Part print with two shaded views. Sizes in mm from the minimum x, y, z corner. A direction names the side the tool comes from. Give positions to 0.01 mm unless a question says otherwise; leave off trailing zeros. Write each loop counter-clockwise with the first axis right and the second up, starting at its lowest first coordinate (ties: lowest second). Pieces come first, ordered by that corner, then holes. Notation, with made-up numbers: (55.25, 49.25) -> (86.25, 49.25) arc R15 cw to (86.25, 59.25) -> close; hole circle Ø1 at (9.5, 10.5). An arc over 180 degrees is marked (long way). Write item = value, one per line. Start each with the question number.
Q1. Saw through at C-C, the plane z = 3.5. List the corners of the cut face in (x, y), then the cut area to 3 significant figures.
Q2. Saw through at A-A, the plane x = 6. List the corners of the cut face in (y, z).
Q3. Drop flat-ended pins along their axis: P1, Ø3, axis at x = 4.5, z = 1, coming from the -Y side; P2, Ø2, axis at x = 8.5, z = 0.5, coming from the -Y side. Give the stop position or say it passes through.
Q4. Wall check: line 1 (Y direction, x = 6, z = 2.35); line 2 (Y direction, x = 6, z = 0.8); line 3 (Z direction, x = 2, y = 1.75). Give the ranges that are in metal, low to high.
Q5. Tool access for the marked faces 1 and 2: list every direction of +Z, -Z, +X, -X, +Y, -Y with a clear straight run to the whole face (end or side of a thin tool).
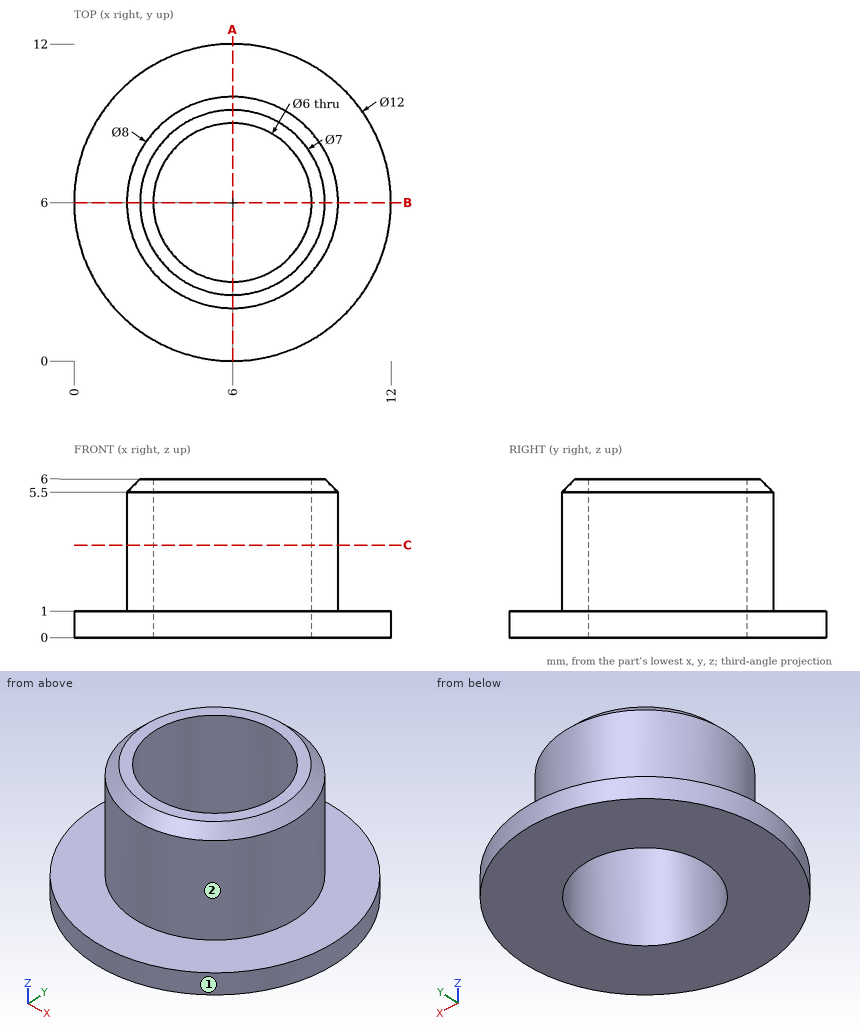
Report:
q1.outline = circle Ø8 at (6, 6); hole circle Ø6 at (6, 6)
q1.area = 22.0 mm2
q2.outline = (0, 0) -> (3, 0) -> (3, 6) -> (2.5, 6) -> (2, 5.5) -> (2, 1) -> (0, 1) -> close; (9, 0) -> (12, 0) -> (12, 1) -> (10, 1) -> (10, 5.5) -> (9.5, 6) -> (9, 6) -> close
q3.P1 = 0
q3.P2 = 0.19
q4.line_1 = 2 to 3, 9 to 10
q4.line_2 = 0 to 3, 9 to 12
q4.line_3 = 0 to 1
q5.face_1 = +Z, -Z
q5.face_2 = +Z
